```python
from build123d import *

# Parameters (mm, degrees)
SKETCH2_R          = 17
CUT_EXTRUDE1_DEPTH = 3


with BuildPart() as part:
    # Sketch1 → Revolve1 (revolve)
    with BuildSketch(Plane(origin=(0, 0, 0), x_dir=(1, 0, 0), z_dir=(0, 1, 0))):
        with BuildLine():
            Line((16, 0), (25.4, 0))
            Line((25.4, 0), (25.4, 2.825))
            ThreePointArc((25.4, 2.825), (22.225, 6), (25.4, 9.175))
            Line((25.4, 9.175), (25.4, 12))
            Line((25.4, 12), (16, 12))
            Line((16, 12), (16, 0))
        make_face()
    revolve(axis=Axis((0, 0, 0), (0, 0, -1)))

    # Sketch2 → Cut-Extrude1 (cut)
    with BuildSketch(Plane(origin=(0, 0, -12), x_dir=(-1, 0, 0), z_dir=(0, 0, -1))):
        Circle(SKETCH2_R)
    extrude(amount=-CUT_EXTRUDE1_DEPTH, mode=Mode.SUBTRACT)


solid = part.part
```
Verification items for the finished model (mm, model axes). Round coordinates to 2 decimals unless told otherwise and drop trailing zeros. Order: outer loops, then holes, each group sorted by start corner. A loop starts at its lowest first (then second) coordinate and runs counter-clockwise, first axis right, second up. Notation, with made-up numbers: (-8.75, 67) - (32.25, 67) arc R23 ccw to (32.25, 80) - close; hole circle Ø11 at (-19.75, 82.5). An arc over 180 degrees is marked (long way). Use CSV: the item, a comma, the result in double quotes.
(1) Mould release check, pull along Y, two halves, no side actions. Record for faces 1 (the face through (0, 17, 0)), 2 (the face through (-9.139, 14.334, -10.521)), 3 (the face through (-5.506, 24.796, -10.607)), 4 (the face through (-13, -10, -9)): released by +Y, released by -Y, zero draft, split by the parting line, or undercut.
Entries:
face 1,"zero draft"
face 2,"undercut"
face 3,"split by the parting line"
face 4,"undercut"
(2) Thickness scan on probe 1 along X at (y, z) = (0, -2.75); probe 2 along Y at (x, z) = (0, -10.2); probe 3 along X at (y, z) = (8, -4). Record the ranges inside material, lowest first. Write a range as from..to.
Entries:
probe 1,"-25.4..-16, 16..25.4"
probe 2,"-25.4..-17, 17..25.4"
probe 3,"-21.49..-13.86, 13.86..21.49"
(3) Section check A-A on x = 0. Record the boundary of the cut face in (y, z) (3 decimals), and give its area (3 significant figures).
Entries:
outline,"(-25.4, -12) - (-17, -12) - (-17, -9) - (-16, -9) - (-16, 0) - (-25.4, 0) - (-25.4, -2.825) arc R3.175 cw to (-25.4, -9.175) - close; (16, -9) - (17, -9) - (17, -12) - (25.4, -12) - (25.4, -9.175) arc R3.175 cw to (25.4, -2.825) - (25.4, 0) - (16, 0) - close"
area,"188 mm^2"
(4) Gauge pin test, flat ends, axial feed: pin 1 Ø1.5 at (x, z) = (-2.5, -7) entering from -Y; pin 2 Ø1.5 at (y, z) = (-4.5, -3) entering from -X; pin 3 Ø8 at (x, y) = (10, 8) entering from -Z. Record the tip position at first contact, or that the pin passes through.
Entries:
pin 1,"y = -22.62"
pin 2,"x = -25.12"
pin 3,"z = -9"
(5) Section check C-C on z = -10.5. Record the boundary of the cut face in (x, y), and give its area (3 significant figures).
Entries:
outline,"circle Ø50.8 at (0, 0); hole circle Ø34 at (0, 0)"
area,"1,120 mm^2"
